Geometry: final body of the model. Coordinates: model frame, mm. A direction names the side the tool comes from. Give positions to 0.01 mm unless a question says otherwise; leave off trailing zeros. Order: outer loops, then holes, each group sorted by start corner. A loop starts at its lowest first (then second) coordinate and runs counter-clockwise, first axis right, second up. Notation, with made-up numbers: M -16,-27 L 39,-27 A26 ccw 39,-7 Z; hole C 30,34.25 d11. An arc over 180 degrees is marked long. One line per item, written item: value. Start each with the question number.
```python
from build123d import *

# Parameters (mm, degrees)
F1_DEPTH = 12.7
F2_R     = 6.35
F3_DEPTH = 12.7
F4_R     = 12.7
F5_DEPTH = 25.4


with BuildPart() as f1:
    # F0 (on Top) → F1 (new body)
    with BuildSketch(Plane.XY):
        with BuildLine():
            ThreePointArc((-56.690635, -28.497916), (-52.970891, -37.478172), (-43.990635, -41.197916))
            Line((-43.990635, -41.197916), (57.609365, -41.197916))
            ThreePointArc((57.609365, -41.197916), (66.589621, -37.478172), (70.309365, -28.497916))
            Line((70.309365, -28.497916), (70.309365, 22.302084))
            Line((70.309365, 22.302084), (-56.690635, 22.302084))
            Line((-56.690635, 22.302084), (-56.690635, -28.497916))
        make_face()
    extrude(amount=F1_DEPTH)

    # F2 (on face) → F3 (cut)
    with BuildSketch(Plane.XY.offset(12.7)):
        with Locations((-37.640635, -25.535107)):
            Circle(F2_R)
        with Locations((51.259365, -25.535107)):
            Circle(F2_R)
        with Locations((51.259365, 3.252084)):
            Circle(F2_R)
    extrude(amount=-F3_DEPTH, mode=Mode.SUBTRACT)

    # F4 (on face) → F5 (join)
    with BuildSketch(Plane(origin=(0, 22.302084, 0), x_dir=(-1, 0, 0), z_dir=(0, 1, 0))):
        with BuildLine():
            Line((5.890635, 63.5), (5.890635, 38.1))
            ThreePointArc((5.890635, 38.1), (-1.548853, 20.139488), (-19.509365, 12.7))
            Line((-19.509365, 12.7), (56.690635, 12.7))
            Line((56.690635, 12.7), (56.690635, 63.5))
            ThreePointArc((56.690635, 63.5), (31.290635, 88.9), (5.890635, 63.5))
        make_face()
        with Locations((31.290635, 63.5)):
            Circle(F4_R, mode=Mode.SUBTRACT)
    extrude(amount=-F5_DEPTH)


solid = f1.part
```
Q1. Contact query for flat-ended pins moving along their axis: pin 1 (11.5 mm diameter, centred on x = 51.26, y = 3.25, fed in from -Z); pin 2 (20.5 mm diameter, centred on x = -37.64, y = -25.54, fed in from +Z); pin 3 (1.5 mm diameter, centred on x = -26, z = 77.5, fed in from -Y); pin 4 (12.5 mm diameter, centred on y = 8, z = 49, fed in from +X). Output: stop coordinate, or through.
Q2. Ray query, line 1 along Y through (x, z) = (53, 11.5); line 2 along Z through (x, y) = (51, 14.5); line 3 along X through (y, z) = (-1, 55.5). Return the intervals inside material, ascending. Write a range as [from, to].
Q3. Set-up query: faces 1 (the face through (-5.891, 10, 51)), 2 (the face through (-35, -3.098, 43)), 3 (the face through (20, -16, 12.7)), 4 (the face through (6, -41.198, 6)). Return all of +Z, -Z, +X, -X, +Y, -Y with unobstructed straight access to the full face (end or side cutting, diameter ignored); none if empty.
Q4. Section query A-A on y = 11.5. Return loops of the section in (x, z), and give its area (3 significant figures).
Q5. Section query B-B on x = 47. Return loops of the section in (y, z), and give its area (3 significant figures).
Q6. Section query D-D on y = -11. Return loops of the section in (x, z), and give its area (3 significant figures).
Q7. Mould query, pull axis Z, two halves, no side actions, for faces 5 (the face through (1.35, 9.78, 20.34)), 6 (the face through (-39.017, -31.734, 6.439)), 7 (the face through (-18.603, 9.78, 64.058)). Classes: +Z half, -Z half, draft (parallel to the pull), parting line (faces both ways), or undercut.
Q8. Section query C-C on z = 49. Return loops of the section in (x, y).
Results below:
1. pin 1: through
1. pin 2: z = 12.7
1. pin 3: y = -3.1
1. pin 4: x = -5.89
2. line 1: [-41.2, -31.64], [-19.43, -2.85], [9.36, 22.3]
2. line 2: [0, 12.7]
2. line 3: [-56.69, -41.15], [-21.43, -5.89]
3. face 1: +Z, +X, +Y, -Y
3. face 2: +Z, +X, -X, -Y
3. face 3: +Z, +X, -Y
3. face 4: +Z, -Z, +X, -X, -Y
4. outline: M -56.69,0 L 70.31,0 L 70.31,12.7 L 19.51,12.7 A25.4 cw -5.89,38.1 L -5.89,63.5 A25.4 ccw -56.69,63.5 Z; hole C -31.29,63.5 d25.4
4. area: 4,840 mm2
5. outline: M -41.2,0 L -30.24,0 L -30.24,12.7 L -41.2,12.7 Z; M -20.83,0 L -1.46,0 L -1.46,12.7 L -20.83,12.7 Z; M 7.96,0 L 22.3,0 L 22.3,12.7 L 7.96,12.7 Z
5. area: 567 mm2
6. outline: M -56.69,0 L 70.31,0 L 70.31,12.7 L -56.69,12.7 Z
6. area: 1,610 mm2
7. face 5: +Z half
7. face 6: draft
7. face 7: undercut
8. outline: M -56.69,-3.1 L -5.89,-3.1 L -5.89,22.3 L -56.69,22.3 Z
